from build123d import *

# Parameters (mm, degrees)
BOSS_EXTRUDE1_DEPTH = 0.5
BOSS_EXTRUDE2_DEPTH = 3.18
SKETCH4_R           = 0.215
BOSS_EXTRUDE3_DEPTH = 13.2
FILLET5_R           = 0.1
FILLET6_R           = 0.1


with BuildPart() as part:
    # Sketch1 → Boss-Extrude1 (new body)
    with BuildSketch(Plane.XY):
        with BuildLine():
            Line((-3.175, 2.5), (3.175, 2.5))
            ThreePointArc((3.175, 2.5), (5.675, 0), (3.175, -2.5))
            Line((3.175, -2.5), (-3.175, -2.5))
            ThreePointArc((-3.175, -2.5), (-5.675, 0), (-3.175, 2.5))
        make_face()
    extrude(amount=-BOSS_EXTRUDE1_DEPTH)

    # Sketch3 → Boss-Extrude2 (add)
    with BuildSketch(Plane(origin=(0, 0, -0.5), x_dir=(-1, 0, 0), z_dir=(0, 0, -1))):
        with BuildLine():
            Line((-3.25, 1.9), (3.25, 1.9))
            ThreePointArc((3.25, 1.9), (5.15, 0), (3.25, -1.9))
            Line((3.25, -1.9), (-3.25, -1.9))
            ThreePointArc((-3.25, -1.9), (-5.15, 0), (-3.25, 1.9))
        make_face()
    extrude(amount=BOSS_EXTRUDE2_DEPTH)

    # Sketch4 → Boss-Extrude3 (add)
    with BuildSketch(Plane.XY):
        with Locations((-2.44, 0)):
            Circle(SKETCH4_R)
        with Locations((2.44, 0)):
            Circle(SKETCH4_R)
    extrude(amount=BOSS_EXTRUDE3_DEPTH)

    # Fillet5
    fillet5_edges = [part.edges().sort_by_distance(p)[0] for p in [
        (5.15, 0, -3.68),
        (0, -1.9, -3.68),
        (-5.15, 0, -3.68),
        (0, 1.9, -3.68),
    ]]
    fillet(fillet5_edges, radius=FILLET5_R)

    # Fillet6
    fillet6_edges = [part.edges().sort_by_distance(p)[0] for p in [
        (5.675, 0, -0.5),
        (0, 2.5, -0.5),
        (-5.675, 0, -0.5),
        (0, -2.5, -0.5),
    ]]
    fillet(fillet6_edges, radius=FILLET6_R)


solid = part.part
Verification items for the finished model (mm, model axes). A direction names the side the tool comes from. Coordinates: 2 decimals unless noted, no trailing zeros. Loops run counter-clockwise (first coordinate to the right, second up) from the corner with the lowest first, then second, coordinate; pieces in that order, holes last. Notation, with made-up numbers: M -29,49.5 L -4,49.5 A25 cw -4,74.5 Z; hole C 3.5,23 d6. An arc over 180 degrees is marked long. One line per item, written item: value.
1. Set-up check for faces 1 (the flat face through (0, -1.9, -2)), 2 (the flat face through (0, 1.9, -2)), 3 (the cylindrical face through (5.15, -0.04, -2.02)), 4 (the cylindrical face through (-5.15, 0.04, -2.02)): record each of +Z, -Z, +X, -X, +Y, -Y from which the full face is reachable in a straight line by a thin tool's end or side.
Answers follow:
face 1: -Z, +X, -X, -Y
face 2: -Z, +X, -X, +Y
face 3: -Z, +X
face 4: -Z, -X
2. Gauge pin test, flat ends, axial feed: P1, Ø1, axis at x = 1, z = 7, coming from the +Y side; P2, Ø1.5, axis at x = 4.5, y = 0, coming from the +Z side; P3, Ø4, axis at x = 1.5, z = 6, coming from the -Y side (3 decimals); P4, Ø1.5, axis at x = 1, z = -2, coming from the +Y side. Record the tip position at first contact, or that the pin passes through.
Answers follow:
P1: through
P2: z = 0
P3: y = -0.215
P4: y = 1.9
3. Section check D-D on z = -1.25. Record the cut outline in (x, y).
Answers follow:
outline: M -3.25,-1.9 L 3.25,-1.9 A1.9 ccw 3.25,1.9 L -3.25,1.9 A1.9 ccw Z
4. Section check B-B on z = 5. Record the cut outline in (x, y) (3 decimals), plus the area to 3 significant figures.
Answers follow:
outline: C -2.44,0 d0.43; C 2.44,0 d0.43
area: 0.290 mm^2
5. Material ranges on line 1 along Z through (x, y) = (3, 1.8); line 2 along Z through (x, y) = (4.75, 1.4); line 3 along Y through (x, z) = (4.75, -1), recorded low to high. Write a range as from..to.
Answers follow:
line 1: -3.68..0
line 2: -0.5..0
line 3: -1.17..1.17
6. Section check C-C on y = 0. Record the cut outline in (x, z) (3 decimals).
Answers follow:
outline: M -5.675,-0.4 A0.1 ccw -5.575,-0.5 L -5.15,-0.5 L -5.15,-3.58 A0.1 ccw -5.05,-3.68 L 5.05,-3.68 A0.1 ccw 5.15,-3.58 L 5.15,-0.5 L 5.575,-0.5 A0.1 ccw 5.675,-0.4 L 5.675,0 L 2.655,0 L 2.655,13.2 L 2.225,13.2 L 2.225,0 L -2.225,0 L -2.225,13.2 L -2.655,13.2 L -2.655,0 L -5.675,0 Z
7. Section check A-A on x = 3. Record the cut outline in (y, z).
Answers follow:
outline: M -2.5,-0.4 A0.1 ccw -2.4,-0.5 L -1.9,-0.5 L -1.9,-3.58 A0.1 ccw -1.8,-3.68 L 1.8,-3.68 A0.1 ccw 1.9,-3.58 L 1.9,-0.5 L 2.4,-0.5 A0.1 ccw 2.5,-0.4 L 2.5,0 L -2.5,0 Z
